Build history of the part. All positions in model axes, mm. Give positions to 0.01 mm unless a question says otherwise; leave off trailing zeros. Loops run counter-clockwise (first coordinate to the right, second up) from the corner with the lowest first, then second, coordinate; pieces in that order, holes last. Notation, with made-up numbers: M -6.5,39.25 L 31.5,39.25 A15 ccw 31.5,64.25 Z; hole C 53,62.25 d7. An arc over 180 degrees is marked long. Answer as a JSON object with one key per item and string values. Group by question number.
1. Mould opens along X. For faces 1 (the face through (14.623, -4.431, -6.063)), 2 (the face through (-12.49, -17.62, 11.46)), 3 (the face through (-14, -21.02, 8)) say: released by +X, released by -X, zero draft, split by the parting line, or undercut.
2. Slice it at D-D (y = -6.5). List the corners of the cut face in (x, z).
3. Drop flat-ended pins along their axis: pin 1 Ø19 at (x, z) = (0, 0) entering from -Y; pin 2 Ø5 at (x, z) = (-0.5, 15) entering from +Y; pin 3 Ø5 at (x, y) = (-5, -11.5) entering from +Z; pin 4 Ø12 at (x, y) = (4.5, 8.5) entering from -Z. Give the stop position or say it passes through.
4. Slice it at B-B (z = 0). List the corners of the cut face in (x, y), then the cut area to 3 significant figures.
5. Slice it at A-A (x = 0). List the corners of the cut face in (y, z), then the cut area to 3 significant figures.
6. Slice it at C-C (y = 2.5). List the corners of the cut face in (x, z).
7. Drill centre lines: line 1 along Z through (x, y) = (0, -2.5); line 2 along X through (y, z) = (-10.5, 4.5); line 3 along X through (y, z) = (-12, 14.5). Where is each one in solid material? Low to high. Write a range as [from, to].
from build123d import *

# Parameters (mm, degrees)
F2_R     = 16.95
F3_DEPTH = 21.02
F4_R     = 15.83
F5_DEPTH = 50
F6_W     = 7.37
F6_H     = 60
F7_DEPTH = 50


with BuildPart() as f1:
    # F0 (on Right) → F1 (revolve)
    with BuildSketch(Plane.YZ):
        with BuildLine():
            Line((-22.18, 0), (22.18, 0))
            ThreePointArc((22.18, 0), (0, 22.18), (-22.18, 0))
        make_face()
    revolve(axis=Axis((0, 3.1962443806, 0), (0, 1, 0)))

    # F2 (on Front) → F3 (join)
    with BuildSketch(Plane.XZ):
        Circle(F2_R)
    extrude(amount=F3_DEPTH)

    # F4 (on face) → F5 (cut, symmetric)
    with BuildSketch(Plane.XZ.offset(21.02)):
        Circle(F4_R)
    extrude(amount=F5_DEPTH, both=True, mode=Mode.SUBTRACT)

    # F6 (on Right) → F7 (cut, symmetric)
    with BuildSketch(Plane.YZ):
        with Locations((16.315, 0)):
            Rectangle(F6_W, F6_H)
    extrude(amount=F7_DEPTH, both=True, mode=Mode.SUBTRACT)


solid = f1.part
Established:
{
 "1": {"face 1": "undercut", "face 2": "split by the parting line", "face 3": "zero draft"},
 "2": {"outline": "C 0,0 d42.41; hole C 0,0 d31.66"},
 "3": {"pin 1": "passes through", "pin 2": "stops at y = 12.63", "pin 3": "stops at z = 19.78", "pin 4": "stops at z = -21.88"},
 "4": {"outline": "M -18.23,12.63 A22.18 ccw -16.95,-14.31 L -16.95,-21.02 L -15.83,-21.02 L -15.83,12.63 Z; M 15.83,-21.02 L 16.95,-21.02 L 16.95,-14.31 A22.18 ccw 18.23,12.63 L 15.83,12.63 Z", "area": "278 mm^2"},
 "5": {"outline": "M -21.02,-16.95 L -14.31,-16.95 A22.18 ccw 12.63,-18.23 L 12.63,-15.83 L -21.02,-15.83 Z; M -21.02,15.83 L 12.63,15.83 L 12.63,18.23 A22.18 ccw -14.31,16.95 L -21.02,16.95 Z", "area": "278 mm^2"},
 "6": {"outline": "C 0,0 d44.08; hole C 0,0 d31.66"},
 "7": {"line 1": "z = [-22.04, -15.83], [15.83, 22.04]", "line 2": "x = [-19.01, -15.18], [15.18, 19.01]", "line 3": "x = [-11.73, -6.35], [6.35, 11.73]"}
}
